```python
from build123d import *

# Parameters (mm, degrees)
F0_R     = 77.2459494585
F1_DEPTH = 152.4
F2_T     = -2.54


# Not quite as in the source:
# - a fillet or chamfer that OpenCascade refuses, or shapes differently, is made with other operations: its cross-section is extruded or revolved along the edge and cut away or added


with BuildPart() as f1:
    # F0 (on Top) → F1 (new body)
    with BuildSketch(Plane.XY):
        Circle(F0_R)
    extrude(amount=F1_DEPTH)

    # F2
    f2_openings = [f1.faces().sort_by_distance(p)[0] for p in [
        (0, 0, 152.4),
    ]]
    offset(amount=F2_T, openings=f2_openings)

    # F3: fillet of radius 5.08 on 3 edges, made by hand

    # F3_s1 → F3_t2 (revolve, cut)
    with BuildSketch(Plane.XZ):
        with BuildLine():
            ThreePointArc((77.2459494585, 5.08), (75.758051907, 1.4878975516), (72.1659494585, 0))
            Line((72.1659494585, 0), (72.1659494585, -0.1016))
            Line((72.1659494585, -0.1016), (77.3475494585, -0.1016))
            Line((77.3475494585, -0.1016), (77.3475494585, 5.08))
            Line((77.3475494585, 5.08), (77.2459494585, 5.08))
        make_face()
    revolve(axis=Axis((0, 0, 0), (0, 0, 1)), mode=Mode.SUBTRACT)

    # F3_s3 → F3_t4 (revolve, cut)
    with BuildSketch(Plane.XZ):
        with BuildLine():
            ThreePointArc((77.2459494585, 148.0005909488), (76.5653585098, 150.5405909488), (74.7059494585, 152.4))
            Line((74.7059494585, 152.4), (74.7567494585, 152.487988181))
            ThreePointArc((74.7567494585, 152.487988181), (75.9759494585, 152.5016), (77.2459494585, 152.5016))
            Line((77.2459494585, 152.5016), (77.3475494585, 152.4))
            Line((77.3475494585, 152.4), (77.3475494585, 148.0005909488))
            Line((77.3475494585, 148.0005909488), (77.2459494585, 148.0005909488))
        make_face()
    revolve(axis=Axis((0, 0, 152.4), (0, 0, 1)), mode=Mode.SUBTRACT)


solid = f1.part
```
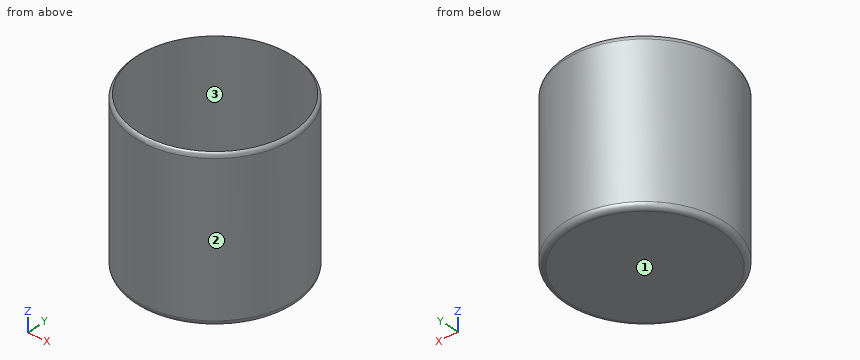
Work out the finished part from the listing and answer in its coordinate system (mm). Face numbers are marked on the shaded views. Give positions to 0.01 mm unless a question says otherwise; leave off trailing zeros. Loops run counter-clockwise (first coordinate to the right, second up) from the corner with the lowest first, then second, coordinate; pieces in that order, holes last. Notation, with made-up numbers: (4.25, 12.5) - (43.25, 12.5) arc R24 cw to (43.25, 30.5) - close; hole circle Ø6 at (-22.75, 85.25). An arc over 180 degrees is marked (long way). One line per question, with ' | ' between items.
(1) Straight lines are drawn through the part: probe 1 along Y at (x, z) = (0, 102); probe 2 along Z at (x, y) = (2.5, 2); probe 3 along Y at (x, z) = (-39, 135). For each, find the intervals that lie inside material, in ascending order.
Recorded:
probe 1: y = -77.25 to -74.71, 74.71 to 77.25 | probe 2: z = 0 to 2.54 | probe 3: y = -66.68 to -63.72, 63.72 to 66.68
(2) The part is cut by section A-A (x = 0). Write down the section's boundary in (y, z), then the cut area to 3 significant figures.
Recorded:
outline: (-77.25, 5.08) arc R5.08 ccw to (-72.17, 0) - (72.17, 0) arc R5.08 ccw to (77.25, 5.08) - (77.25, 148) arc R5.08 ccw to (74.71, 152.4) - (74.71, 2.54) - (-74.71, 2.54) - (-74.71, 152.4) arc R5.08 ccw to (-77.25, 148) - close | area: 1,140 mm²
(3) The mould has two halves that part along X. Classify the marked faces 1, 2 and 3: +X half, -X half, draft (parallel to the pull), parting line (faces both ways), or undercut.
Recorded:
face 1: draft | face 2: parting line | face 3: undercut
(4) Each of these flat-tipped pins is pushed along its axis until it touches: pin 1 Ø6 at (x, z) = (-35.5, 69) entering from +Y; pin 2 Ø4 at (y, z) = (8.5, 63) entering from -X; pin 3 Ø1 at (y, z) = (-10, 47.5) entering from -X. Where does it stop, or does it pass through?
Recorded:
pin 1: stops at y = 70.08 | pin 2: stops at x = -76.97 | pin 3: stops at x = -76.66
(5) The part is cut by section C-C (z = 33). Write down the section's boundary in (x, y), then the cut area to 3 significant figures.
Recorded:
outline: circle Ø154.49 at (0, 0); hole circle Ø149.41 at (0, 0) | area: 1,210 mm²
